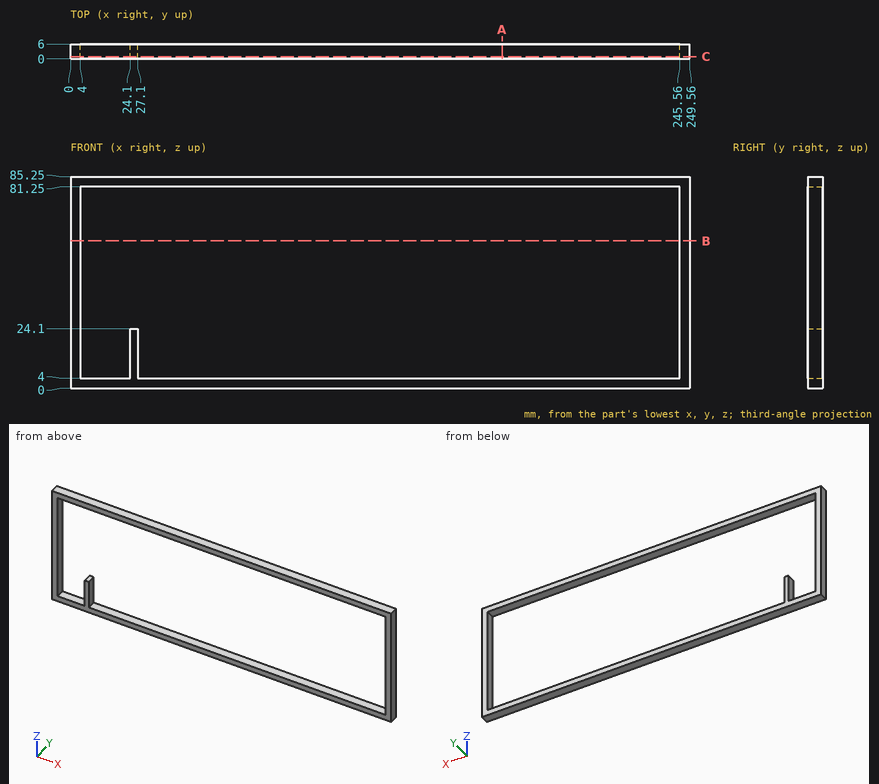
Geometry: see drawing. Coordinates: mm, zero at the bounding-box minimum. Coordinates: 2 decimals unless noted, no trailing zeros. Loops run counter-clockwise (first coordinate to the right, second up) from the corner with the lowest first, then second, coordinate; pieces in that order, holes last. Notation, with made-up numbers: M 5,33 L 48,33 A26 cw 48,48 Z; hole C 56,68.25 d6. An arc over 180 degrees is marked long. Answer in a Markdown table with one row per item.
1. Section B-B, the plane z = 59.5. Output: boundary loops of the cut face in (x, y), then the cut area to 3 significant figures.
Response:
| item | result |
|---|---|
| outline | M 0,0 L 4,0 L 4,6 L 0,6 Z; M 245.56,0 L 249.56,0 L 249.56,6 L 245.56,6 Z |
| area | 48.0 mm2 |
2. Section C-C, the plane y = 0.95. Output: boundary loops of the cut face in (x, z), then the cut area to 3 significant figures.
Response:
| item | result |
|---|---|
| outline | M 0,0 L 249.56,0 L 249.56,85.25 L 0,85.25 Z; hole M 4,4 L 24.1,4 L 24.1,24.1 L 27.1,24.1 L 27.1,4 L 245.56,4 L 245.56,81.25 L 4,81.25 Z |
| area | 2,670 mm2 |
3. First-contact query: pin 1 (10 mm diameter, centred on x = 125, z = 75, fed in from +Y). Flat tip, straight axial feed; report the tip coordinate or a pass-through.
Response:
| item | result |
|---|---|
| pin 1 | passes through |
4. Material intervals for line 1 (X direction, y = 3.75, z = 13); line 2 (Z direction, x = 165, y = 0.5); line 3 (X direction, y = 3.8, z = 45.5), sorted ascending.
Response:
| item | result |
|---|---|
| line 1 | x = 0 to 4, 24.1 to 27.1, 245.56 to 249.56 |
| line 2 | z = 0 to 4, 81.25 to 85.25 |
| line 3 | x = 0 to 4, 245.56 to 249.56 |
5. Section A-A, the plane x = 174. Output: boundary loops of the cut face in (y, z), then the cut area to 3 significant figures.
Response:
| item | result |
|---|---|
| outline | M 0,0 L 6,0 L 6,4 L 0,4 Z; M 0,81.25 L 6,81.25 L 6,85.25 L 0,85.25 Z |
| area | 48.0 mm2 |
